Design review of the part shown in the three views and the two pictorial views. Dimensions are in mm from the part's minimum x, y and z. Give positions to 0.01 mm unless a question says otherwise; leave off trailing zeros. Loops run counter-clockwise (first coordinate to the right, second up) from the corner with the lowest first, then second, coordinate; pieces in that order, holes last. Notation, with made-up numbers: (49, -28.75) - (61, -28.75) arc R23 ccw to (61, -11.75) - close; hole circle Ø5 at (58, 39.5). An arc over 180 degrees is marked (long way). Put each result on its own line as item: value. Start each with the question number.
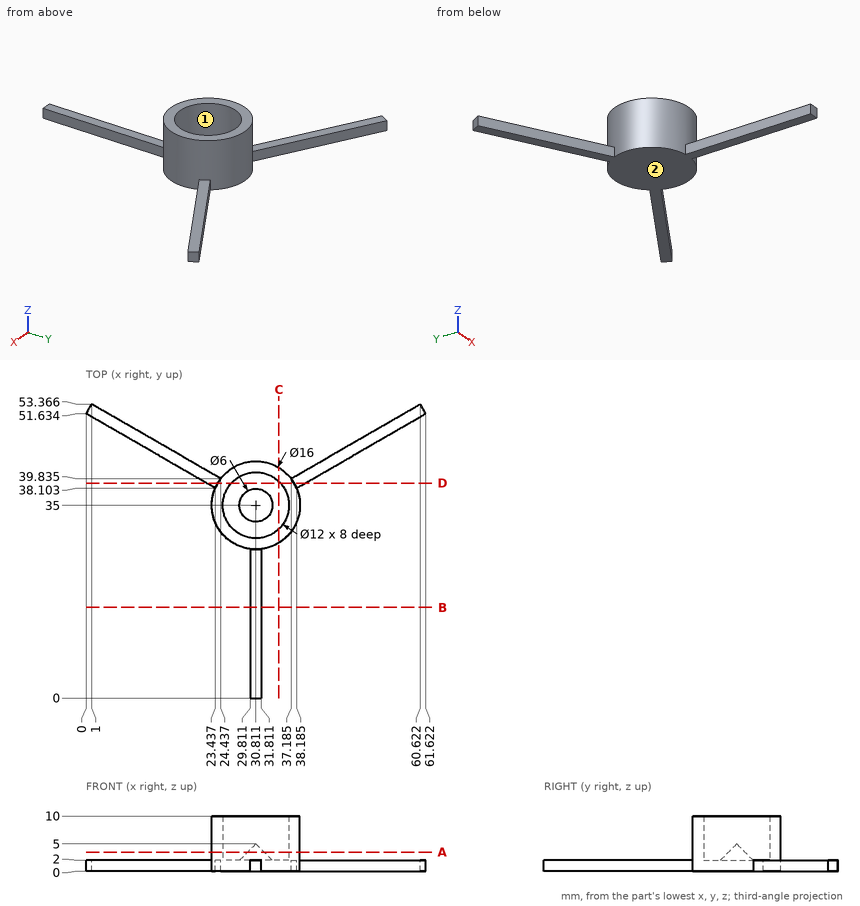
1) Take a section at A-A on z = 3.5. State the section outline as (x, y) points.
2) Take a section at B-B on y = 16.5. State the section outline as (x, z) points.
3) Take a section at C-C on x = 35. State the section outline as (y, z) points (1 decimal).
4) Mouldability with a two-part tool opening along Y and no side actions: class the marked faces 1 and 2 as released by +Y, released by -Y, zero draft, split by the parting line, or undercut.
5) Insertion check: P1, Ø5, axis at y = 36, z = 8.5, coming from the +X side; P2, Ø3.5, axis at x = 28.5, y = 32, coming from the +Z side; P3, Ø1, axis at y = 20, z = 0.5, coming from the +X side. Each pin has a flat end and moves straight along its axis. Give the tip position at first contact, or say it passes through.
6) Wall thickness on probe 1 along Y at (x, z) = (33, 2.5) (1 decimal); probe 2 along X at (y, z) = (35, 5.75); probe 3 along Y at (x, z) = (30.5, 9.75): over which ranges is each line inside the solid? List them lowest first.
7) Take a section at D-D on y = 39. State the section outline as (x, z) points.
Answers follow:
1. outline: circle Ø16 at (30.81, 35); circle Ø3 at (30.81, 35); hole circle Ø12 at (30.81, 35)
2. outline: (29.81, 0) - (31.81, 0) - (31.81, 2) - (29.81, 2) - close
3. outline: (28.2, 0) - (41.8, 0) - (41.8, 10) - (39.3, 10) - (39.3, 2) - (30.7, 2) - (30.7, 10) - (28.2, 10) - close
4. face 1: undercut
4. face 2: zero draft
5. P1: x = 38.81
5. P2: z = 2.96
5. P3: x = 31.81
6. probe 1: 27.3 to 29.4, 33.8 to 36.2, 40.6 to 42.7
6. probe 2: 22.81 to 24.81, 36.81 to 38.81
6. probe 3: 27.01 to 29.01, 40.99 to 42.99
7. outline: (21.88, 0) - (39.74, 0) - (39.74, 2) - (37.74, 2) - (37.74, 10) - (35.28, 10) - (35.28, 2) - (26.34, 2) - (26.34, 10) - (23.88, 10) - (23.88, 2) - (21.88, 2) - close
